Check sheet for the drawn part. Datum: minimum x, y, z corner. Units: mm. A direction names the side the tool comes from. Coordinates: 2 decimals unless noted, no trailing zeros. Loops run counter-clockwise (first coordinate to the right, second up) from the corner with the lowest first, then second, coordinate; pieces in that order, holes last. Notation, with made-up numbers: (-27, 0.5) - (24, 0.5) arc R19 cw to (24, 13.5) - close; hole circle Ø3 at (37.5, 44). An arc over 180 degrees is marked (long way). Answer as a JSON object with one key per item and string values. Group by question number.
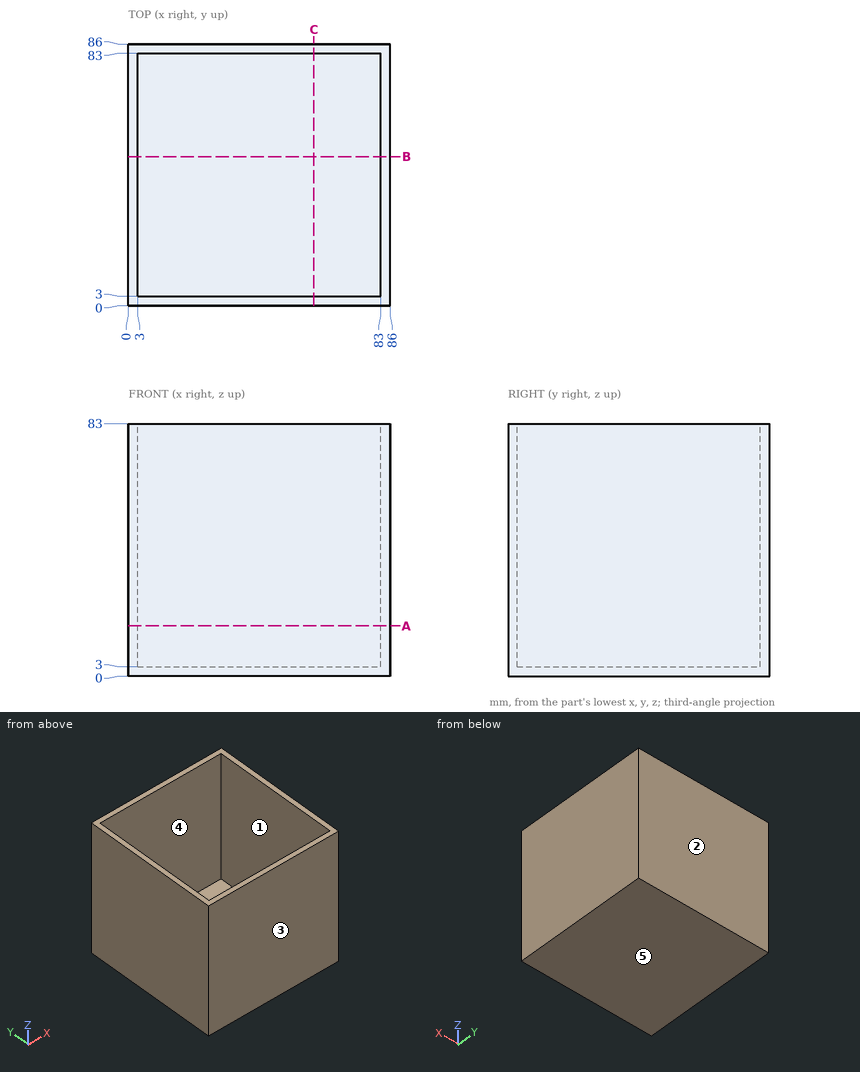
1. Access from +Z, -Z, +X, -X, +Y, -Y to the whole of each face (thin tool, end or side, straight path). Record for the marked faces 1 and 2.
2. Release check for a two-part mould opening along Y. For the marked faces 3, 4 and 5 record: released by +Y, released by -Y, zero draft, split by the parting line, or undercut.
3. Sectioned sample at B-B on y = 49. Record the cut outline in (x, z), plus the area to 3 significant figures.
4. Material ranges on line 1 (X direction, y = 57.5, z = 26.5); line 2 (Z direction, x = 43.5, y = 43), recorded low to high.
5. Sectioned sample at A-A on z = 16.5. Record the cut outline in (x, y), plus the area to 3 significant figures.
6. Gauge pin test, flat end, axial feed: pin 1 (5 mm diameter, centred on x = 72.5, y = 63.5, fed in from +Z). Record the tip position at first contact, or that the pin passes through.
Answers follow:
{
 "1": {"face 1": "+Z", "face 2": "+Z, -Z, +X, -X, +Y"},
 "2": {"face 3": "released by -Y", "face 4": "undercut", "face 5": "zero draft"},
 "3": {"outline": "(0, 0) - (86, 0) - (86, 83) - (83, 83) - (83, 3) - (3, 3) - (3, 83) - (0, 83) - close", "area": "738 mm^2"},
 "4": {"line 1": "x = 0 to 3, 83 to 86", "line 2": "z = 0 to 3"},
 "5": {"outline": "(0, 0) - (86, 0) - (86, 86) - (0, 86) - close; hole (3, 3) - (83, 3) - (83, 83) - (3, 83) - close", "area": "996 mm^2"},
 "6": {"pin 1": "stops at z = 3"}
}
